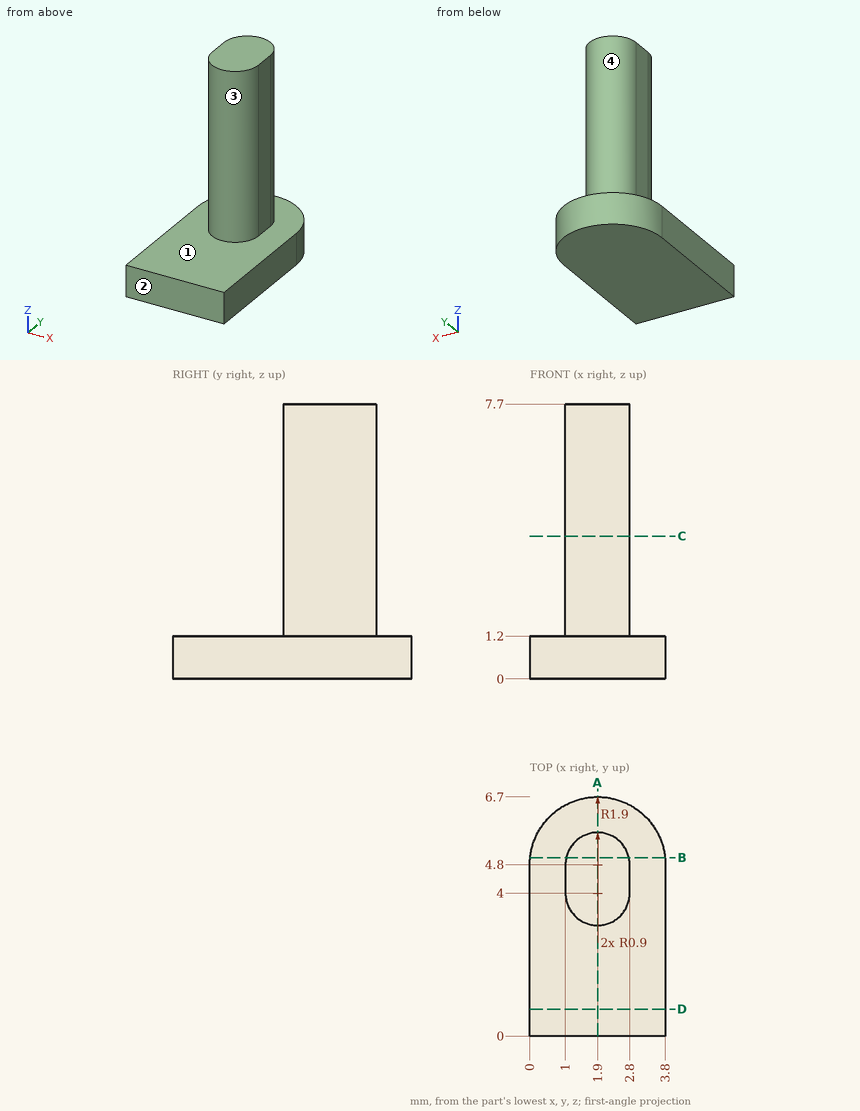
Could you check a few things on this drawing? It's one solid part, dimensions in mm from its lowest x, y, z. A direction names the side the tool comes from. Round coordinates to 2 decimals unless told otherwise and drop trailing zeros. Loops run counter-clockwise (first coordinate to the right, second up) from the corner with the lowest first, then second, coordinate; pieces in that order, holes last. Notation, with made-up numbers: (17.5, 14.25) -> (53.5, 14.25) arc R24 cw to (53.5, 50.25) -> close; hole circle Ø7 at (46.25, 75.25). An arc over 180 degrees is marked (long way). One line per item, written item: value. Start each with the question number.
1. For pin 1 (0.6 mm diameter, centred on y = 4.5, z = 3.5, fed in from -X); pin 2 (1.5 mm diameter, centred on x = 0.5, z = 4.5, fed in from -Y); pin 3 (1 mm diameter, centred on x = 2, z = 3, fed in from -Y), each with a flat end and sliding along its axis, tell me the tip position at first contact or that it passes through.
2. If we section it at D-D, the plane y = 0.75: Write out the boundary of the cut face in (x, z).
3. If I drill on probe 1 along X at (y, z) = (4.25, 5); probe 2 along Z at (x, y) = (2.2, 2); probe 3 along Y at (x, z) = (1.85, 7.5), over which ranges is the centre line in solid material (lowest first)?
4. If we section it at B-B, the plane y = 5: Write out the boundary of the cut face in (x, z), then the cut area to 3 significant figures.
5. If we section it at C-C, the plane z = 4: Write out the boundary of the cut face in (x, y).
6. For the marked faces 1, 2, 3 and 4, which set-ups out of +Z, -Z, +X, -X, +Y, -Y let a thin tool reach every point of the face, with its end or its side?
7. If we section it at A-A, the plane x = 1.9: Write out the boundary of the cut face in (y, z).
Calculated:
1. pin 1: stops at x = 1
1. pin 2: stops at y = 3.38
1. pin 3: stops at y = 3.1
2. outline: (0, 0) -> (3.8, 0) -> (3.8, 1.2) -> (0, 1.2) -> close
3. probe 1: x = 1 to 2.8
3. probe 2: z = 0 to 1.2
3. probe 3: y = 3.1 to 5.7
4. outline: (0.01, 0) -> (3.79, 0) -> (3.79, 1.2) -> (2.78, 1.2) -> (2.78, 7.7) -> (1.02, 7.7) -> (1.02, 1.2) -> (0.01, 1.2) -> close
4. area: 15.9 mm²
5. outline: (1, 4) arc R0.9 ccw to (2.8, 4) -> (2.8, 4.8) arc R0.9 ccw to (1, 4.8) -> close
6. face 1: +Z
6. face 2: +Z, -Z, +X, -X, -Y
6. face 3: +Z, -Y
6. face 4: +Z, +Y
7. outline: (0, 0) -> (6.7, 0) -> (6.7, 1.2) -> (5.7, 1.2) -> (5.7, 7.7) -> (3.1, 7.7) -> (3.1, 1.2) -> (0, 1.2) -> close
